Source: CAD feature listing. Evaluate the final solid. Frame: model axes, mm. Give positions to 0.01 mm unless a question says otherwise; leave off trailing zeros. Loops run counter-clockwise (first coordinate to the right, second up) from the corner with the lowest first, then second, coordinate; pieces in that order, holes last.
from build123d import *

# Parameters (mm, degrees)
ESBO_O1_R                  = 1.75
RESSALTO_EXTRUS_O1_DEPTH   = 3
ESBO_O2_W                  = 30
ESBO_O2_H                  = 3
RESSALTO_EXTRUS_O2_DEPTH   = 43
CORTE_EXTRUS_O1_DEPTH      = 61.613529843
CORTE_EXTRUS_O1_DEPTH_BACK = 61.613529843
ESBO_O4_R                  = 1.75
CORTE_EXTRUS_O2_DEPTH      = 61.613529843


with BuildPart() as part:
    # Esboço1 → Ressalto-extrusão1 (new body)
    with BuildSketch(Plane.XY):
        with BuildLine():
            Line((-15, 11.357178844), (-15, -13.642821156))
            Line((-15, -13.642821156), (15, -13.642821156))
            Line((15, -13.642821156), (15, 11.357178844))
            ThreePointArc((15, 11.357178844), (0, 26.357178844), (-15, 11.357178844))
        make_face()
        with Locations((0, 11.357178844)):
            Circle(ESBO_O1_R, mode=Mode.SUBTRACT)
    extrude(amount=RESSALTO_EXTRUS_O1_DEPTH)

    # Esboço2 → Ressalto-extrusão2 (add)
    with BuildSketch(Plane(origin=(0, 0, 0), x_dir=(-1, 0, 0), z_dir=(0, 0, -1))):
        with Locations((0, -15.142821156)):
            Rectangle(ESBO_O2_W, ESBO_O2_H)
    extrude(amount=-RESSALTO_EXTRUS_O2_DEPTH)

    # Esboço3 → Corte-extrusão1 (cut, two sides: drawn at the far end of the back side and taken through both)
    with BuildSketch(Plane(origin=(0, -13.642821156, 0), x_dir=(1, 0, 0), z_dir=(0, 1, 0)).offset(-CORTE_EXTRUS_O1_DEPTH_BACK)):
        with BuildLine():
            Line((15, -43), (15, -28))
            ThreePointArc((15, -28), (10.606601736, -38.606601699), (5.3e-08, -43))
            Line((5.3e-08, -43), (15, -43))
        make_face()
        with BuildLine():
            Line((-15, -43), (5.3e-08, -43))
            ThreePointArc((5.3e-08, -43), (-10.606601699, -38.606601736), (-15, -28))
            Line((-15, -28), (-15, -43))
        make_face()
    extrude(amount=CORTE_EXTRUS_O1_DEPTH + CORTE_EXTRUS_O1_DEPTH_BACK, mode=Mode.SUBTRACT)

    # Esboço4 → Corte-extrusão2 (cut, through all)
    with BuildSketch(Plane(origin=(0, -13.642821156, 0), x_dir=(1, 0, 0), z_dir=(0, 1, 0))):
        with Locations(Location((0, -28, 0), (0, 0, 270))):
            Circle(ESBO_O4_R)
    extrude(amount=-CORTE_EXTRUS_O2_DEPTH, mode=Mode.SUBTRACT)


solid = part.part
1) Cut plane A-A (y = 12.5). Return loops of the section in (x, z), and give its area (3 significant figures).
Checks:
outline: (-14.96, 0) - (-1.33, 0) - (-1.33, 3) - (-14.96, 3) - close; (1.33, 0) - (14.96, 0) - (14.96, 3) - (1.33, 3) - close
area: 81.8 mm2
2) Contact query for flat-ended pins moving along their axis: P1, Ø4, axis at x = 0, y = 7, coming from the +Z side; P2, Ø5, axis at x = -1.5, y = 20, coming from the -Z side; P3, Ø5, axis at x = 2.5, z = 27, coming from the +Y side; P4, Ø3, axis at x = 0, z = 28, coming from the +Y side. Output: stop coordinate, or through.
Checks:
P1: stops at z = 3
P2: stops at z = 0
P3: stops at y = -13.64
P4: passes through
3) Cut plane B-B (z = 37). Return loops of the section in (x, y).
Checks:
outline: (-12, -16.64) - (12, -16.64) - (12, -13.64) - (-12, -13.64) - close
4) Cut plane C-C (x = -8.25). Return loops of the section in (y, z), and give its area (3 significant figures).
Checks:
outline: (-16.64, 0) - (23.88, 0) - (23.88, 3) - (-13.64, 3) - (-13.64, 40.53) - (-16.64, 40.53) - close
area: 234 mm2
5) Pull-direction query (Y, two-part tool) for faces 1 (the cylindrical face through (-0.23, 13.09, 1.48)), 2 (the flat face through (0, 7, 3)), 3 (the flat face through (0, -13.643, 23)), 4 (the flat face through (0, -16.643, 21)); classes: released by +Y, released by -Y, zero draft, split by the parting line, or undercut.
Checks:
face 1: undercut
face 2: zero draft
face 3: released by +Y
face 4: released by -Y
6) Cut plane D-D (y = -11). Return loops of the section in (x, z).
Checks:
outline: (-15, 0) - (15, 0) - (15, 3) - (-15, 3) - close
7) Ray query, probe 1 along Y at (x, z) = (0, 0.7); probe 2 along Y at (x, z) = (-3.75, 35); probe 3 along Z at (x, y) = (8, -8.5). Return the intervals inside material, ascending.
Checks:
probe 1: y = -16.64 to 9.61, 13.11 to 26.36
probe 2: y = -16.64 to -13.64
probe 3: z = 0 to 3
